Part model, mm, in its own coordinate system. Face numbers are marked on the shaded views. A direction names the side the tool comes from. Round coordinates to 2 decimals unless told otherwise and drop trailing zeros. Loops run counter-clockwise (first coordinate to the right, second up) from the corner with the lowest first, then second, coordinate; pieces in that order, holes last. Notation, with made-up numbers: (-26, -10.75) -> (-17, -10.75) arc R28 ccw to (-17, 18.25) -> close; hole circle Ø11 at (-13.75, 35). An arc over 180 degrees is marked (long way). Use a Markdown table: item, result. Add a question column.
Item 1: Two-plate mould, pull along Y, no slides. Class the marked faces 3, 4 and 5: pulls with the +Y half, pulls with the -Y half, needs draft (parallel to the pull), parting line crosses it, or undercut.
Item 2: Which spindle directions (+Z, -Z, +X, -X, +Y, -Y) get a long thin tool onto all of the face, cutting with end or side? Do the marked faces 1 and 2. Say none if no direction does.
Item 3: Flat gauge pins, fed straight in: pin 1 (15 mm diameter, centred on y = 20, z = -846.5, fed in from +X); pin 2 (5 mm diameter, centred on y = 15.5, z = -816.5, fed in from +X). Where does each tip first touch, or does it go through?
Item 4: Cut at C-C, the plane x = 20.5. List the corners of the cut face in (y, z) (3 decimals).
Item 5: Cut at A-A, the plane z = -800.1. List the corners of the cut face in (x, y) (3 decimals), plus the area to 3 significant figures.
Item 6: Cut at D-D, the plane y = 21. List the corners of the cut face in (x, z).
Item 7: Cut at B-B, the plane z = -787.4. List the corners of the cut face in (x, y) (3 decimals), plus the area to 3 significant figures.
Item 8: Probe line 1 (Y direction, x = 8, z = -792) (3 decimals); line 2 (X direction, y = 22, z = -847); line 3 (X direction, y = 1, z = -800). List the from-to ranges inside material, lowest first. Write a range as [from, to].
Autodesk Inventor part; units mm, degrees
ref_plane "YZ Plane" through (0, 0, 0) normal (1, 0, 0) x (0, 1, 0)
ref_plane "XZ Plane" through (0, 0, 0) normal (0, 1, 0) x (-1, 0, 0)
ref_plane "XY Plane" through (0, 0, 0) normal (0, 0, 1) x (1, 0, 0)
sketch "Sketch1" plane through (0, 0, 0) normal (0, 0, 1) x (1, 0, 0)
  line L0 (5.9771, 0) -> (28.2021, 0)
  line L1 (28.2021, 0) -> (28.2021, 3.175)
  line L2 (28.2021, 3.175) -> (5.9771, 3.175)
  line L3 (2.8021, 6.35) -> (2.8021, 25.4)
  line L4 (5.9771, 28.575) -> (28.2021, 28.575)
  line L5 (28.2021, 28.575) -> (28.2021, 31.75)
  line L6 (28.2021, 31.75) -> (5.9771, 31.75)
  line L7 (-0.3729, 25.4) -> (-0.3729, 6.35)
  arc A0 (5.9771, 28.575) -> (2.8021, 25.4) centre (5.9771, 25.4) ccw
  arc A1 (2.8021, 6.35) -> (5.9771, 3.175) centre (5.9771, 6.35) ccw
  arc A2 (5.9771, 31.75) -> (-0.3729, 25.4) centre (5.9771, 25.4) ccw
  arc A3 (-0.3729, 6.35) -> (5.9771, 0) centre (5.9771, 6.35) ccw
  point P0 (0, 0)
  point P1 (-0.3729, 0)
  point P2 (2.8021, 3.175)
  point P3 (2.8021, 28.575)
  dimension "d0" = 28.575
  dimension "d1" = 3.175
  dimension "d2" = 25.4
  dimension "d3" = 25.4
  dimension "d4" = 3.175
  dimension "d5" = 3.175
  dimension "d6" = 6.35
extrude "Extrusion1" add sketch "Sketch1" against normal blind 889
sketch "Sketch2" plane through (-0.3729, 6.35, 0) normal (-1, 0, 0) x (0, 0, 1)
  line L0 (0, 19.05) -> (-889, 19.05)
  line L1 (-228.6, 0) -> (-228.6, 7.9375)
  arc A0 (-228.6, 11.1125) -> (-228.6, 7.9375) centre (-228.6, 9.525) ccw
  line L2 (-228.6, 11.1125) -> (-228.6, 19.05)
  line L3 (-228.6, 19.05) -> (-889, 19.05)
  line L4 (-889, 0) -> (-889, 19.05)
  line L5 (-889, 0) -> (-228.6, 0)
  circle A1 centre (-552.45, 11.43) radius 4.826
  circle A2 centre (-501.65, 11.43) radius 4.826
  circle A3 centre (-387.35, 11.43) radius 4.826
  circle A4 centre (-336.55, 11.43) radius 4.826
  circle A5 centre (-444.5, 7.62) radius 4.826
  circle A6 centre (-730.25, 11.43) radius 4.826
  circle A7 centre (-781.05, 11.43) radius 4.826
  line L6 (0, 25.4) -> (-889, 25.4) construction
  circle A8 centre (-133.35, 11.43) radius 4.826
  circle A9 centre (-82.55, 11.43) radius 4.826
  point P0 (0, -6.35)
  point P1 (-254, 0.852)
  dimension "d10" = 7.62
  dimension "d11" = 3.81
  dimension "d14" = 254
hole "Hole1" at (-0.3729, 17.78, -781.05) at (-0.3729, 17.78, -730.25) at (-0.3729, 17.78, -552.45) at (-0.3729, 17.78, -501.65) at (-0.3729, 13.97, -444.5) at (-0.3729, 17.78, -387.35) at (-0.3729, 17.78, -336.55) at (-0.3729, 17.78, -133.35) at (-0.3729, 17.78, -82.55) direction (1, 0, 0) diameter 9.652 end through all
hole "Hole2" at (-0.3729, 15.875, -228.6) direction (1, 0, 0) diameter 3.175 end through all
sketch "Sketch3" plane through (5.9771, 31.75, 0) normal (0, 1, 0) x (1, 0, 0)
  line L0 (22.225, 889) -> (0, 889)
  line L1 (22.225, 0) -> (22.225, 889)
  point P0 (-5.9771, 0)
  point P1 (9.525, 876.3)
  dimension "d34" = 12.7
  dimension "d35" = 12.7
hole "Hole3" at (15.5021, 31.75, -876.3) direction (0, -1, 0) diameter 6.5278 end through all
pattern_linear "Rectangular Pattern1" count 35 spacing 25.4 along (0, 0, 1) of "Hole3"
sketch "Sketch4" plane through (0, 0, 0) normal (0, 0, 1) x (1, 0, 0)
  line L0 (28.2021, 0) -> (5.9771, 0)
  line L1 (28.2021, 3.175) -> (28.2021, 0)
  line L2 (5.9771, 3.175) -> (28.2021, 3.175)
  arc A0 (2.8021, 6.35) -> (5.9771, 3.175) centre (5.9771, 6.35) ccw
  line L3 (2.8021, 25.4) -> (2.8021, 6.35)
  arc A1 (5.9771, 28.575) -> (2.8021, 25.4) centre (5.9771, 25.4) ccw
  line L4 (28.2021, 28.575) -> (5.9771, 28.575)
  line L5 (28.2021, 31.75) -> (28.2021, 28.575)
  line L6 (5.9771, 31.75) -> (28.2021, 31.75)
  arc A2 (5.9771, 31.75) -> (-0.3729, 25.4) centre (5.9771, 25.4) ccw
  line L7 (-0.3729, 6.35) -> (-0.3729, 25.4)
  arc A3 (-0.3729, 6.35) -> (5.9771, 0) centre (5.9771, 6.35) ccw
  point P0 (0, 0)
extrude "Extrusion2" cut sketch "Sketch4" against normal blind 774.7
sketch "Sketch5" plane through (15.5021, 3.175, -774.7) normal (0, 1, 0) x (1, 0, 0)
  circle A0 centre (0.1108, 85.1274) radius 3.5719
  circle A1 centre (0.1108, 85.1274) radius 14.2875 construction
  point P0 (-15.5021, -774.7)
extrude "Extrusion3" cut sketch "Sketch5" against normal through all
ref_plane "Work Plane1" through (28.2021, 31.75, -889) normal (0.6428, 0, -0.766) x (0, 1, 0)
sketch "Sketch6" plane through (28.2021, 31.75, -889) normal (0.6428, 0, -0.766) x (0, 1, 0)
  line L0 (-28.575, 73.4706) -> (-31.75, 73.4706) construction
  line L1 (-31.75, 73.4706) -> (-31.75, 0) construction
  line L2 (-31.75, 0) -> (-28.575, 0) construction
  line L3 (-28.575, 73.4706) -> (-28.575, 0) construction
  line L4 (0, 73.4706) -> (-3.175, 73.4706) construction
  line L5 (-3.175, 73.4706) -> (-3.175, 0) construction
  line L6 (-3.175, 0) -> (0, 0) construction
  line L7 (0, 73.4706) -> (0, 0) construction
  line L8 (-31.75, 0) -> (-28.575, 0)
  line L9 (-31.75, -17.0253) -> (-31.75, 0)
  ellipse E0 centre (-25.4, -17.0253) end of major axis (-19.05, -17.0253) minor radius 4.8644 (-31.75, -17.0253) -> (-25.4, -21.8897) ccw construction
  line L10 (-6.35, -21.8897) -> (-25.4, -21.8897) construction
  ellipse E1 centre (-6.35, -17.0253) end of major axis (-12.7, -17.0253) minor radius 4.8644 (-6.35, -21.8897) -> (0, -17.0253) ccw construction
  line L11 (0, 0) -> (0, -17.0253)
  line L12 (-3.175, 0) -> (0, 0)
  line L13 (-3.175, -17.0253) -> (-3.175, 0) construction
  ellipse E2 centre (-6.35, -17.0253) end of major axis (-3.175, -17.0253) minor radius 2.4322 (-6.35, -19.4575) -> (-3.175, -17.0253) ccw construction
  line L14 (-25.4, -19.4575) -> (-6.35, -19.4575) construction
  ellipse E3 centre (-25.4, -17.0253) end of major axis (-22.225, -17.0253) minor radius 2.4322 (-28.575, -17.0253) -> (-25.4, -19.4575) ccw construction
  line L15 (-28.575, 0) -> (-28.575, -17.0253) construction
  line L16 (-31.75, 19.05) -> (0, 19.05)
  line L17 (0, 19.05) -> (0, -31.75)
  line L18 (0, -31.75) -> (-31.75, -31.75)
  line L19 (-31.75, -31.75) -> (-31.75, 19.05)
  point P0 (-31.75, 549.8341)
  dimension "d54" = 31.75
  dimension "d55" = 50.8
  dimension "d56" = 19.05
extrude "Extrusion4" cut sketch "Sketch6" against normal blind 12.7
sketch "Sketch7" plane through (2.8021, 6.35, -774.7) normal (1, 0, 0) x (0, 0, -1)
  circle A0 centre (6.35, 11.43) radius 4.826
  circle A1 centre (101.6, 9.525) radius 1.5875
  line L0 (6.35, 11.43) -> (101.6, 9.525) construction
  line L1 (114.3, 9.525) -> (101.6, 9.525) construction
  line L2 (114.3, 0) -> (114.3, 19.05)
  point P0 (-774.7, -6.35)
  dimension "d59" = 3.175
  dimension "d60" = 95.269
extrude "Extrusion5" cut sketch "Sketch7" against normal through all contours A1
sketch "Sketch8" plane through (15.5021, 28.575, -774.7) normal (0, -1, 0) x (1, 0, 0)
  circle A0 centre (0, -12.7) radius 3.175
  circle A1 centre (24.765, -101.6) radius 3.175 construction
  circle A2 centre (-24.765, -101.6) radius 3.175 construction
  circle A3 centre (0, -101.6) radius 3.175 construction
  circle A4 centre (-24.765, -12.7) radius 3.175 construction
  circle A5 centre (24.765, -12.7) radius 3.175 construction
  line L0 (-37.465, -111.125) -> (-37.465, -3.175) construction
  line L1 (37.465, -111.125) -> (-37.465, -111.125) construction
  line L2 (37.465, -111.125) -> (37.465, -3.175) construction
  line L3 (-37.465, -3.175) -> (37.465, -3.175) construction
  point P0 (-15.5021, 774.7)
extrude "Extrusion6" cut sketch "Sketch8" against normal through all
properties part number "Chassis_Channel_AndyMark (4.5 inch)"
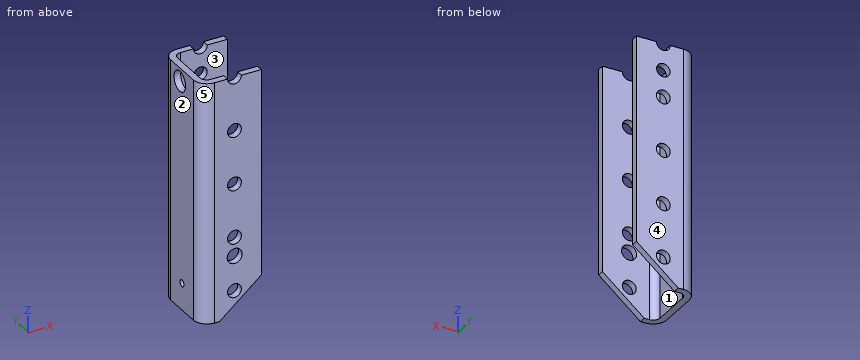
A:
| question | item | result |
|---|---|---|
| 1 | face 3 | undercut |
| 1 | face 4 | pulls with the +Y half |
| 1 | face 5 | pulls with the -Y half |
| 2 | face 1 | +Z, -Z, +X |
| 2 | face 2 | +Z, -Z, -X, +Y, -Y |
| 3 | pin 1 | stops at x = 3.6 |
| 3 | pin 2 | stops at x = 2.8 |
| 4 | outline | (0, -878.882) -> (3.175, -878.882) -> (3.175, -774.7) -> (0, -774.7) -> close; (28.575, -878.882) -> (31.75, -878.882) -> (31.75, -774.7) -> (28.575, -774.7) -> close |
| 5 | outline | (-0.373, 6.35) arc R6.35 ccw to (5.977, 0) -> (12.238, 0) -> (12.238, 3.175) -> (5.977, 3.175) arc R3.175 cw to (2.802, 6.35) -> (2.802, 25.4) arc R3.175 cw to (5.977, 28.575) -> (12.238, 28.575) -> (12.238, 31.75) -> (5.977, 31.75) arc R6.35 ccw to (-0.373, 25.4) -> close; (18.766, 0) -> (28.202, 0) -> (28.202, 3.175) -> (18.766, 3.175) -> close; (18.766, 28.575) -> (28.202, 28.575) -> (28.202, 31.75) -> (18.766, 31.75) -> close |
| 5 | area | 208 mm^2 |
| 6 | outline | (-0.37, -889) -> (2.8, -889) -> (2.8, -784.64) -> (-0.37, -784.64) -> close; (-0.37, -777.46) -> (2.8, -777.46) -> (2.8, -774.7) -> (-0.37, -774.7) -> close |
| 7 | outline | (-0.373, 6.35) arc R6.35 ccw to (5.977, 0) -> (28.202, 0) -> (28.202, 3.175) -> (5.977, 3.175) arc R3.175 cw to (2.802, 6.35) -> (2.802, 25.4) arc R3.175 cw to (5.977, 28.575) -> (12.327, 28.575) -> (12.327, 31.75) -> (5.977, 31.75) arc R6.35 ccw to (-0.373, 25.4) -> close; (18.677, 28.575) -> (28.202, 28.575) -> (28.202, 31.75) -> (18.677, 31.75) -> close |
| 7 | area | 229 mm^2 |
| 8 | line 1 | y = [0, 3.175], [28.575, 31.75] |
| 8 | line 2 | x = [-0.37, 2.8] |
| 8 | line 3 | x = [2.56, 12.24], [18.76, 28.2] |
